Autodesk Inventor part; units mm, degrees
ref_plane "YZ Plane" through (0, 0, 0) normal (1, 0, 0) x (0, 1, 0)
ref_plane "XZ Plane" through (0, 0, 0) normal (0, 1, 0) x (-1, 0, 0)
ref_plane "XY Plane" through (0, 0, 0) normal (0, 0, 1) x (1, 0, 0)
sketch "Sketch1" plane through (0, 0, 0) normal (0, 1, 0) x (-1, 0, 0)
  line L0 (130, 230) -> (-130, 230)
  line L1 (-130, 230) -> (-130, -230)
  line L2 (-130, -230) -> (130, -230)
  line L3 (130, -230) -> (130, 230)
  line L4 (130, 230) -> (-130, -230) construction
  line L5 (-130, 230) -> (130, -230) construction
  line L6 (124.5, -224.5) -> (-124.5, -224.5)
  line L7 (-124.5, -224.5) -> (-124.5, 224.5)
  line L8 (-124.5, 224.5) -> (124.5, 224.5)
  line L9 (124.5, 224.5) -> (124.5, -224.5)
  line L10 (124.5, -224.5) -> (-124.5, 224.5) construction
  line L11 (-124.5, -224.5) -> (124.5, 224.5) construction
  line L12 (-109.5, 209.5) -> (109.5, 209.5)
  line L13 (109.5, 209.5) -> (109.5, -209.5)
  line L14 (109.5, -209.5) -> (-109.5, -209.5)
  line L15 (-109.5, -209.5) -> (-109.5, 209.5)
  line L16 (-109.5, 209.5) -> (109.5, -209.5) construction
  line L17 (109.5, 209.5) -> (-109.5, -209.5) construction
  point P0 (0, 0)
  dimension "d0" = 260
  dimension "d1" = 460
  dimension "d8" = 249
  dimension "d9" = 449
  dimension "d10" = 219
  dimension "d11" = 419
extrude "Extrusion3" add sketch "Sketch1" along normal blind 5 contours L6 L7 L8 L9
equation "\"d0\" = boxl + 2 * pvct"
equation "\"d1\" = boxw + 2 * pvct"
equation "\"d8\" = boxl - 2 * play"
equation "\"d9\" = boxw - 2 * play"
equation "\"d10\" = boxl - 2 * play - 2 * supporth"
equation "\"d11\" = boxw - 2 * play - 2 * supporth"
equation "\"d12\" = pvct"
equation "\"solhole\" = 3"
equation "\"solholespacing\" = 16"
equation "\"ssolw\" = 63"
equation "\"bsoll\" = 126"
equation "\"bsolw\" = 91"
equation "\"bsolh\" = 126"
equation "\"tapl\" = 31"
equation "\"tl\" = 32"
equation "\"eloboww\" = 25"
equation "\"pvct\" = 5"
equation "\"boxh\" = 258"
equation "\"supporth\" = 15"
equation "\"play\" = 0.5"
equation "\"arw\" = 54"
equation "\"arl\" = 102"
equation "\"psuh\" = 85"
equation "\"screenw\" = 197"
equation "\"screenl\" = 115"
equation "\"pcbw\" = 76"
equation "\"pcbl\" = 86"
equation "\"pcbh\" = 46"
equation "\"seph\" = 105"
equation "\"diaetape\" = 25"
equation "\"diaload\" = 16"
equation "\"diapower\" = 16"
equation "\"diaph\" = 32"
equation "\"distbubblewater\" = 82"
equation "\"distpumps\" = 75"
equation "\"waterouter\" = 39"
equation "\"waterinner\" = 28"
equation "\"pumpinner\" = 16"
equation "\"pumpouter\" = 25"
equation "\"airoutinner\" = 28"
equation "\"airoutouter\" = 39"
equation "\"airinouter\" = 39"
equation "\"airininner\" = 28"
equation "\"diapowerouter\" = 25"
equation "\"dialoadouter\" = 25"
equation "\"diaetapeouter\" = 36"
equation "\"diaphouter\" = 48"
properties part number "sb_bottom" material "PVC-Piping"
Build history of the part. All positions in model axes, mm. Coordinates: 2 decimals unless noted, no trailing zeros. Order: outer loops, then holes, each group sorted by start corner. A loop starts at its lowest first (then second) coordinate and runs counter-clockwise, first axis right, second up. Notation, with made-up numbers: M 38.25,28 L 81.25,28 A14 cw 81.25,52 Z; hole C 70.5,13 d9. An arc over 180 degrees is marked long. One line per question, with ' | ' between items. Start each with the question number.
1. Cut at C-C (z = 149.5). Write the cut outline in (x, y), plus the area to 3 significant figures.
2. Cut at B-B (y = 3.6). Write the cut outline in (x, z), plus the area to 3 significant figures.
3. Wall check: line 1 along X through (y, z) = (3.1, 7); line 2 along Z through (x, y) = (87.5, 3.2). Give the ranges that are in metal, low to high. Write a range as [from, to].
4. Cut at A-A (x = -82.5). Write the cut outline in (y, z).
The answers:
1) outline: M -124.5,0 L -109.5,0 L -109.5,5 L -124.5,5 Z; M 109.5,0 L 124.5,0 L 124.5,5 L 109.5,5 Z | area: 150 mm2
2) outline: M -124.5,-224.5 L 124.5,-224.5 L 124.5,224.5 L -124.5,224.5 Z; hole M -109.5,-209.5 L 109.5,-209.5 L 109.5,209.5 L -109.5,209.5 Z | area: 20,000 mm2
3) line 1: x = [-124.5, -109.5], [109.5, 124.5] | line 2: z = [-224.5, -209.5], [209.5, 224.5]
4) outline: M 0,-224.5 L 5,-224.5 L 5,-209.5 L 0,-209.5 Z; M 0,209.5 L 5,209.5 L 5,224.5 L 0,224.5 Z
